```python
from build123d import *

# Parameters (mm, degrees)
SKETCH1_R           = 15
BOSS_EXTRUDE2_DEPTH = 145
BOSS_EXTRUDE3_START = 50
SKETCH5_R           = 5
BOSS_EXTRUDE3_DEPTH = 20
SHELL1_START        = -125
SHELL1_DEPTH        = 250
SKETCH6_W           = 520
SKETCH6_H           = 290
BOSS_EXTRUDE4_DEPTH = 20
FILLET1_R           = 20


# Read off the part's stored shape, not the designer's step: Shell1
with BuildPart() as part:
    # Sketch1 → Boss-Extrude2 (new, symmetric)
    with BuildSketch(Plane.XY):
        with BuildLine():
            Line((0, 120), (0, 0))
            Line((0, 0), (520, 0))
            Line((520, 0), (520, 120))
            Line((520, 120), (414.127591904, 178.329519311))
            ThreePointArc((414.127591904, 178.329519311), (390.743657055, 184.530618142), (367.18562851, 179.027770991))
            Line((367.18562851, 179.027770991), (262.81437149, 125.508377715))
            ThreePointArc((262.81437149, 125.508377715), (251.734966676, 121.396599326), (240, 120))
            Line((240, 120), (0, 120))
        make_face()
        with Locations((390, 140)):
            Circle(SKETCH1_R, mode=Mode.SUBTRACT)
    extrude(amount=BOSS_EXTRUDE2_DEPTH, both=True)

    # Sketch5 → Boss-Extrude3 (add)
    with BuildSketch(Plane.XY.offset(BOSS_EXTRUDE3_START)):
        with BuildLine():
            Line((240, 120), (0, 120))
            Line((0, 120), (0, 204))
            ThreePointArc((0, 204), (12.346331353, 222.47759065), (34.142135624, 218.142135624))
            Line((34.142135624, 218.142135624), (122.284271247, 130))
            Line((122.284271247, 130), (271.573743284, 130))
            Line((271.573743284, 130), (262.81437149, 125.508377715))
            ThreePointArc((262.81437149, 125.508377715), (251.734966676, 121.396599326), (240, 120))
        make_face()
        with Locations((20, 204)):
            Circle(SKETCH5_R, mode=Mode.SUBTRACT)
        with Locations((45, 179)):
            Circle(SKETCH5_R, mode=Mode.SUBTRACT)
    extrude(amount=-BOSS_EXTRUDE3_DEPTH)

    # Mirror1: part across plane


with BuildPart() as part_1:
    add(part.part)
    add(part.part.mirror(Plane.XY))

    # Shell1 outline → Shell1 (cut)
    with BuildSketch(Plane.XY.offset(SHELL1_START)):
        with BuildLine():
            Line((356.85957207, 151.256644109), (271.940120086, 107.711728801))
            ThreePointArc((271.940120086, 107.711728801), (256.428953346, 101.955239056), (240, 100))
            Line((240, 100), (20, 100))
            Line((20, 100), (20, 0))
            Line((20, 0), (500, 0))
            Line((500, 0), (500, 108.184326651))
            Line((500, 108.184326651), (423.428190104, 150.370926015))
            ThreePointArc((423.428190104, 150.370926015), (389.534354317, 105.00309765), (356.85957207, 151.256644109))
        make_face()
    extrude(amount=SHELL1_DEPTH, mode=Mode.SUBTRACT)

    # Sketch6 → Boss-Extrude4 (add)
    # profile 1 of 2: a face of its own
    with BuildSketch(Plane.XZ):
        with Locations((260, 0)):
            Rectangle(SKETCH6_W, SKETCH6_H)
        Polygon((20, 125), (500, 125), (500, -125), (240, -125), (20, -125), align=None, mode=Mode.SUBTRACT)
    # profile 2 of 2: a face of its own
    with BuildSketch(Plane.XZ):
        Polygon((540, 165), (0, 165), (0, 145), (520, 145), (520, -145), (0, -145), (0, -165), (540, -165), align=None)
    extrude(amount=-BOSS_EXTRUDE4_DEPTH)

    # Fillet1
    fillet1_edges = [part_1.edges().sort_by_distance(p)[0] for p in [
        (120, 120, -145),
        (467.063795952, 149.164759656, 145),
        (390.743657055, 184.530618142, 145),
        (315, 152.268074353, 145),
        (251.734966676, 121.396599326, 145),
        (120, 120, 145),
        (251.734966676, 121.396599326, -145),
        (315, 152.268074353, -145),
        (390.743657055, 184.530618142, -145),
        (467.063795952, 149.164759656, -145),
    ]]
    fillet(fillet1_edges, radius=FILLET1_R)


solid = part_1.part
```
Part model, mm, in its own coordinate system. A direction names the side the tool comes from. Round coordinates to 2 decimals unless told otherwise and drop trailing zeros. Order: outer loops, then holes, each group sorted by start corner. A loop starts at its lowest first (then second) coordinate and runs counter-clockwise, first axis right, second up. Notation, with made-up numbers: M 50.25,73.5 L 92.25,73.5 A23 cw 92.25,82.5 Z; hole C -10,30.25 d9. An arc over 180 degrees is marked long. Answer in a Markdown table with one row per item. Add a question column.
Q1. Cut at A-A on z = -37.5. Give the cut face in (x, y).
Q2. 3-axis set-ups, long thin cutter, end or side, ignore diameter. For faces 4 (the face through (77.596, 174.688, -40.14)), 5 (the face through (122, 120, 0)), 6 (the face through (251.896, 121.436, -86.975)): which of +Z, -Z, +X, -X, +Y, -Y reach the whole face in a straight line?
Q3. Cut at D-D on y = 140. Give the number of separate pieces and of enclosed holes in the cut face, and give its area (3 significant figures).
Q4. Cut at C-C on x = 113.5. Give the cut face in (y, z).
Q5. Wall check: L1, parallel to X at y = 31.5, z = -93.5; L2, parallel to Z at x = 455.5, y = 18.5; L3, parallel to Z at x = 196.5, y = 43.5. Give the ranges that are in metal, low to high. Write a range as from..to.
Q6. Pin check, flat tips, straight feed: pin 1 (1.5 mm diameter, centred on y = 38, z = 80, fed in from +X); pin 2 (22 mm diameter, centred on x = 182, z = 35.5, fed in from +Y); pin 3 (6 mm diameter, centred on x = 20, y = 204, fed in from -Z); pin 4 (18 mm diameter, centred on x = 170, z = 1.5, fed in from +Y). Stop position of each tip, or through.
Q7. Cut at B-B on y = 83. Give the cut face in (x, z), and give its area (3 significant figures).
Q8. Mould opens along Z. For faces 1 (the face through (76, 157, 50)), 2 (the face through (390, 105, -2)), 3 (the face through (77.596, 174.688, 40.14)) say: +Z half, -Z half, draft (parallel to the pull), parting line (faces both ways), or undercut.
Established:
| question | item | result |
|---|---|---|
| 1 | outline | M 0,0 L 20,0 L 20,100 L 240,100 A70 ccw 271.94,107.71 L 356.86,151.26 A35 ccw long 423.43,150.37 L 500,108.18 L 500,0 L 540,0 L 540,20 L 520,20 L 520,120 L 414.13,178.33 A50 ccw 367.19,179.03 L 271.57,130 L 122.28,130 L 34.14,218.14 A20 ccw 0,204 Z; hole C 20,204 d10; hole C 45,179 d10; hole C 390,140 d30 |
| 2 | face 4 | +Z, -Z, +Y |
| 2 | face 5 | -X, +Y |
| 2 | face 6 | -Z, -X, +Y |
| 3 | separate pieces | 4 |
| 3 | enclosed holes | 2 |
| 3 | area | 41,600 mm2 |
| 4 | outline | M 0,-165 L 20,-165 L 20,-145 L 100,-145 A20 ccw 120,-125 L 120,-50 L 138.78,-50 L 138.78,-30 L 120,-30 L 120,30 L 138.78,30 L 138.78,50 L 120,50 L 120,125 A20 ccw 100,145 L 20,145 L 20,165 L 0,165 L 0,125 L 100,125 L 100,-125 L 0,-125 Z |
| 5 | L1 | x = 0..20, 500..520 |
| 5 | L2 | z = -165..-125, 125..165 |
| 5 | L3 | z = -145..-125, 125..145 |
| 6 | pin 1 | stops at x = 520 |
| 6 | pin 2 | stops at y = 130 |
| 6 | pin 3 | passes through |
| 6 | pin 4 | stops at y = 120 |
| 7 | outline | M 0,-145 L 520,-145 L 520,145 L 0,145 Z; hole M 20,-125 L 500,-125 L 500,125 L 20,125 Z |
| 7 | area | 30,800 mm2 |
| 8 | face 1 | +Z half |
| 8 | face 2 | undercut |
| 8 | face 3 | draft |
